Source: CAD feature listing. Evaluate the final solid. Frame: model axes, mm. Round coordinates to 2 decimals unless told otherwise and drop trailing zeros. Loops run counter-clockwise (first coordinate to the right, second up) from the corner with the lowest first, then second, coordinate; pieces in that order, holes last.
(1) Material intervals for probe 1 along Z at (x, y) = (483.5, -16.5); probe 2 along Y at (x, z) = (478, -117); probe 3 along X at (y, z) = (-5, -83.5), sorted ascending.
(2) First-contact query: pin 1 Ø1.8 at (x, y) = (492.5, -0.5) entering from +Z; pin 2 Ø3 at (y, z) = (-12, -35.5) entering from -X; pin 3 Ø5 at (x, z) = (500, -16.5) entering from +Y. Flat tips, straight axial feed; report the tip coordinate or a pass-through.
(3) Section A-A, the plane z = -30.5. Return the cut outline in (x, y), plus the area to 3 significant figures.
```python
from build123d import *


with BuildPart() as f1:
    # F0 (on Front) → F1 (revolve)
    with BuildSketch(Plane.XZ):
        with BuildLine():
            Line((489.550671, 7.579802), (489.550671, 8.969648))
            Line((489.550671, 8.969648), (486.550671, 8.969648))
            Line((486.550671, 8.969648), (486.550671, 6.658985))
            Line((486.550671, 6.658985), (480.40905, 6.658985))
            Line((480.40905, 6.658985), (480.40905, 4.440768))
            Line((480.40905, 4.440768), (475.766086, 4.440768))
            Line((475.766086, 4.440768), (475.766086, 5.595956))
            Line((475.766086, 5.595956), (473.550671, 5.595956))
            Line((473.550671, 5.595956), (473.550671, 3.76596))
            ThreePointArc((473.550671, 3.76596), (474.384093, 2.932538), (473.550671, 2.099116))
            Line((473.550671, 2.099116), (473.550671, -122.362282))
            Line((473.550671, -122.362282), (476.530877, -122.362282))
            Line((476.530877, -122.362282), (476.530877, -123.194333))
            Line((476.530877, -123.194333), (486.550671, -124.833937))
            Line((486.550671, -124.833937), (486.550671, -126.030352))
            Line((486.550671, -126.030352), (489.550671, -126.030352))
            Line((489.550671, -126.030352), (489.550671, -122.861977))
            Line((489.550671, -122.861977), (492.550671, -122.861977))
            Line((492.550671, -122.861977), (492.550671, 7.579802))
            Line((492.550671, 7.579802), (489.550671, 7.579802))
        make_face()
    revolve(axis=Axis((492.550671, 0, -54.35379), (0, 0, -1)))


solid = f1.part
```
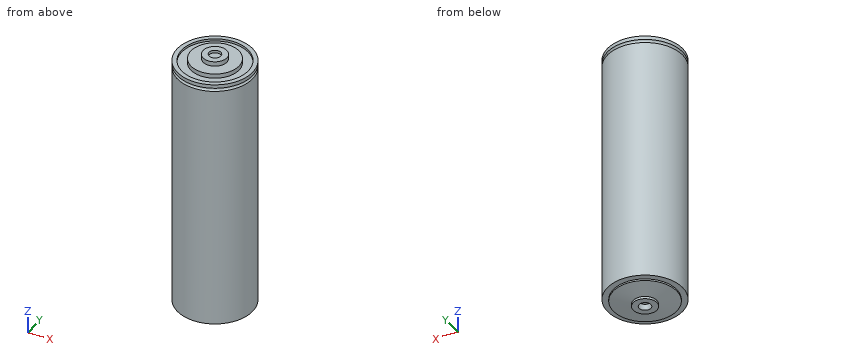
Output values:
1. probe 1: z = -122.36 to 2.12, 3.75 to 5.6
1. probe 2: y = -12.22 to 12.22
1. probe 3: x = 474.22 to 510.88
2. pin 1: stops at z = 7.58
2. pin 2: stops at x = 476.72
2. pin 3: stops at y = 18.34
3. outline: circle Ø38 at (492.55, 0)
3. area: 1,130 mm2
